from build123d import *

# Parameters (mm, degrees)
CUT_EXTRUDE1_DEPTH      = 367.129389697
CUT_EXTRUDE1_DEPTH_BACK = 367.129389697
SKETCH2_W               = 193.8
SKETCH2_H               = 31.1
HOLE1_D                 = 12.5


with BuildPart() as part:
    # Sketch1 → Revolve1 (revolve)
    with BuildSketch(Plane.XY):
        Polygon((0, 0), (0, 20), (28.9, 20), (28.9, 28), (89.3, 28), (89.3, 43.6), (113.3, 43.6), (113.3, 28), (360.9, 28), (360.9, 0), align=None)
    revolve(axis=Axis((360.9, 0, 0), (-1, 0, 0)))

    # Sketch2 → Cut-Extrude1 (cut, two sides: drawn at the far end of the back side and taken through both)
    with BuildSketch(Plane.XY.offset(-CUT_EXTRUDE1_DEPTH_BACK)):
        with Locations((264, 12.45)):
            Rectangle(SKETCH2_W, SKETCH2_H)
    extrude(amount=CUT_EXTRUDE1_DEPTH + CUT_EXTRUDE1_DEPTH_BACK, mode=Mode.SUBTRACT)

    # Hole1 (through all)
    with Locations(Plane(origin=(0, -3.1, 0), x_dir=(1, 0, 0), z_dir=(0, 1, 0))):
        with Locations((199, 0), (299, 0)):
            Hole(HOLE1_D / 2)


solid = part.part
Model file for the job. Use its own axes, mm. A direction names the side the tool comes from. Coordinates: 2 decimals unless noted, no trailing zeros. Write each loop counter-clockwise with the first axis right and the second up, starting at its lowest first coordinate (ties: lowest second). Pieces come first, ordered by that corner, then holes. Notation, with made-up numbers: (61.25, -3) -> (69.25, -3) arc R30 ccw to (69.25, 36) -> close; hole circle Ø10 at (-29.5, -28). An arc over 180 degrees is marked (long way). One line per item, written item: value. Start each with the question number.
1) Slice it at B-B on y = 0. Write the cut outline in (x, z).
2) Slice it at C-C on x = 299. Write the cut outline in (y, z).
3) Pull direction Z, two halves, no side cores. Call faces 5 (the face through (263, -3.1, 0)), 6 (the face through (211.322, -27.973, -1.231)), 7 (the face through (305.244, -15.724, -0.275)): +Z half, -Z half, draft (parallel to the pull), parting line (faces both ways), or undercut.
4) Which spindle directions (+Z, -Z, +X, -X, +Y, -Y) get a long thin tool onto all of the face, cutting with end or side? Do faces 1 (the face through (113.3, -0.6, 28.5)), 2 (the face through (101.468, 41.587, -13.096)), 3 (the face through (167.1, 9, 0)), 4 (the face through (14.652, -4.336, 19.524)). Say none if no direction does.
5) Flat gauge pins, fed straight in: pin 1 Ø3 at (x, z) = (93, -17) entering from -Y; pin 2 Ø12 at (x, z) = (235, -19) entering from +Y; pin 3 Ø7.5 at (x, z) = (299, 0) entering from +Y; pin 4 Ø17 at (y, z) = (4.5, -2.5) entering from -X. Where does each tip first touch, or does it go through?
6) Probe probe 1 along X at (y, z) = (34, 8); probe 2 along X at (y, z) = (0, 12); probe 3 along X at (y, z) = (-25, -5.5). List the from-to ranges inside material, lowest first.
7) Slice it at D-D on y = -16.5. Write the cut outline in (x, z), then the cut area to 3 significant figures.
8) Slice it at A-A on z = 0. Write the cut outline in (x, y).
Answers follow:
1. outline: (0, -20) -> (28.9, -20) -> (28.9, -28) -> (89.3, -28) -> (89.3, -43.6) -> (113.3, -43.6) -> (113.3, -28) -> (167.1, -28) -> (167.1, 28) -> (113.3, 28) -> (113.3, 43.6) -> (89.3, 43.6) -> (89.3, 28) -> (28.9, 28) -> (28.9, 20) -> (0, 20) -> close
2. outline: (-27.29, -6.25) arc R28 ccw to (-3.1, -27.83) -> (-3.1, -6.25) -> close; (-27.29, 6.25) -> (-3.1, 6.25) -> (-3.1, 27.83) arc R28 ccw to start
3. face 5: draft
3. face 6: parting line
3. face 7: undercut
4. face 1: +X
4. face 2: +X, -X
4. face 3: +Z, -Z, +X, +Y
4. face 4: -X
5. pin 1: y = -40.75
5. pin 2: y = -3.1
5. pin 3: through
5. pin 4: x = 0
6. probe 1: 89.3 to 113.3
6. probe 2: 0 to 167.1
6. probe 3: 28.9 to 196.03, 201.97 to 296.03, 301.97 to 360.9
7. outline: (0, -11.3) -> (28.9, -11.3) -> (28.9, -22.62) -> (89.3, -22.62) -> (89.3, -40.36) -> (113.3, -40.36) -> (113.3, -22.62) -> (360.9, -22.62) -> (360.9, 22.62) -> (113.3, 22.62) -> (113.3, 40.36) -> (89.3, 40.36) -> (89.3, 22.62) -> (28.9, 22.62) -> (28.9, 11.3) -> (0, 11.3) -> close; hole circle Ø12.5 at (199, 0); hole circle Ø12.5 at (299, 0)
7. area: 16,300 mm2
8. outline: (0, -20) -> (28.9, -20) -> (28.9, -28) -> (89.3, -28) -> (89.3, -43.6) -> (113.3, -43.6) -> (113.3, -28) -> (192.75, -28) -> (192.75, -3.1) -> (167.1, -3.1) -> (167.1, 28) -> (113.3, 28) -> (113.3, 43.6) -> (89.3, 43.6) -> (89.3, 28) -> (28.9, 28) -> (28.9, 20) -> (0, 20) -> close; (205.25, -28) -> (292.75, -28) -> (292.75, -3.1) -> (205.25, -3.1) -> close; (305.25, -28) -> (360.9, -28) -> (360.9, -3.1) -> (305.25, -3.1) -> close
